Autodesk Inventor part; units mm, degrees
ref_plane "YZ Plane" through (0, 0, 0) normal (1, 0, 0) x (0, 1, 0)
ref_plane "XZ Plane" through (0, 0, 0) normal (0, 1, 0) x (-1, 0, 0)
ref_plane "XY Plane" through (0, 0, 0) normal (0, 0, 1) x (1, 0, 0)
sketch "Sketch1" plane through (0, 0, 0) normal (0, 0, 1) x (1, 0, 0)
  line L0 (-26, -31) -> (26, -31)
  line L1 (26, -31) -> (26, 31)
  line L2 (26, 31) -> (-26, 31)
  line L3 (-26, 31) -> (-26, -31)
  line L4 (-26, -31) -> (26, 31) construction
  line L5 (26, -31) -> (-26, 31) construction
  line L6 (-24, -23) -> (-24, -9) construction
  line L7 (-26, 31) -> (26, 46)
  line L8 (26, 46) -> (86, 46)
  line L9 (86, 46) -> (86, 19)
  line L10 (86, 19) -> (26, 19)
  point P0 (0, 0)
  dimension "d0" = 2
  dimension "d1" = 62
  dimension "d2" = 52
  dimension "d3" = 15
  dimension "d4" = 50
  dimension "d5" = 60
extrude "Extrusion1" add sketch "Sketch1" along normal blind 5
sketch "Sketch2" plane through (0, 0, 5) normal (0, 0, 1) x (1, 0, 0)
  line L0 (-29, 11.5) -> (-29, 6.5) construction
  line L1 (-29, 6.5) -> (-24, 6.5) construction
  line L2 (-24, 6.5) -> (-24, -20) construction
  line L3 (-24, -20) -> (-15, -20) construction
  line L4 (-15, -20) -> (-15, -27) construction
  line L5 (-15, -27) -> (-12, -27) construction
  line L6 (-12, -27) -> (-12, -20) construction
  line L7 (-12, -20) -> (16, -20) construction
  line L8 (16, -20) -> (16, 20) construction
  line L9 (16, 20) -> (11, 20) construction
  line L10 (11, 20) -> (11, 25) construction
  line L11 (11, 25) -> (8, 25) construction
  line L12 (8, 25) -> (8, 20) construction
  line L13 (8, 20) -> (-12, 20) construction
  line L14 (-12, 20) -> (-12, 27) construction
  line L15 (-12, 27) -> (-15, 27) construction
  line L16 (-15, 27) -> (-15, 20) construction
  line L17 (-15, 20) -> (-24, 20) construction
  line L18 (26, 46) -> (-26, 31)
  line L19 (-24, 20) -> (-24, 11.5) construction
  line L20 (-24, 11.5) -> (-29, 11.5) construction
  line L21 (-26, 31) -> (-26, -31) construction
  line L22 (-26, -31) -> (26, -31) construction
  line L23 (-12, 31.0385) -> (-12, 20)
  line L24 (-12, 20) -> (-8, 20)
  line L25 (-8, 20) -> (-8, 32.1923)
  line L26 (-26, 27) -> (26, 42)
  line L27 (-26, -27) -> (-12, -27)
  line L28 (-12, -27) -> (-12, -20)
  line L29 (-12, -20) -> (-8, -20)
  line L30 (-8, -20) -> (-8, -27)
  line L31 (-8, -27) -> (16, -27)
  line L32 (16, -27) -> (16, 20)
  line L33 (26, -31) -> (26, 19)
  line L34 (26, 24) -> (26, 19) construction
  line L35 (-26, 31) -> (-26, 27)
  line L36 (86, 46) -> (26, 46)
  line L37 (26, 46) -> (26, 42)
  line L38 (26, 42) -> (82, 42)
  line L39 (82, 42) -> (82, 19)
  line L40 (26, 19) -> (86, 19)
  line L41 (86, 19) -> (86, 46)
  line L42 (-26, -27) -> (-26, -31)
  line L43 (-26, -31) -> (26, -31)
  line L44 (16, 20) -> (16, 24)
  line L45 (16, 24) -> (26, 24)
  line L46 (26, 24) -> (82, 24)
  line L47 (26, 19) -> (26, 20)
  line L48 (26, 20) -> (82, 20)
  point P0 (0, 0)
  dimension "d8" = 3
  dimension "d9" = 3
  dimension "d10" = 3
  dimension "d11" = 7
  dimension "d12" = 54
  dimension "d13" = 7
  dimension "d14" = 5
  dimension "d15" = 5
  dimension "d16" = 2
  dimension "d17" = 9
  dimension "d18" = 8.5
  dimension "d19" = 4
  dimension "d20" = 5
  dimension "d21" = 5
  dimension "d22" = 40
  dimension "d23" = 4
  dimension "d25" = 4
  dimension "d26" = 10
  dimension "d27" = 4
  dimension "d28" = 4
  dimension "d36" = 1
  dimension "d37" = 4
extrude "Extrusion2" add sketch "Sketch2" along normal blind 10 contours L37 L26 L35 L18 | L36 L41 L40 L39 L38 L37 | L25 L24 L23 L26 | L39 L48 L47 L33 L43 L42 L27 L28 L29 L30 L31 L32 L44 L45 L46
sketch "Sketch3" plane through (0, 0, 15) normal (0, 0, 1) x (1, 0, 0)
  line L0 (-26, 27) -> (-12, 31.0385)
  line L1 (-12, 31.0385) -> (-12, 20)
  line L2 (-12, 20) -> (-8, 20)
  line L3 (-8, 20) -> (-8, 32.1923)
  line L4 (-8, 32.1923) -> (26, 42)
  line L5 (26, 42) -> (82, 42)
  line L6 (82, 42) -> (82, 24)
  line L7 (82, 19) -> (86, 19)
  line L8 (86, 19) -> (86, 46)
  line L9 (86, 46) -> (26, 46)
  line L10 (26, 46) -> (-26, 31)
  line L11 (-26, 31) -> (-26, 27)
  line L12 (30, 42) -> (78, 42)
  line L13 (78, 42) -> (78, 46)
  line L14 (78, 46) -> (30, 46)
  line L15 (30, 46) -> (30, 42)
  line L16 (82, 24) -> (16, 24)
  line L17 (16, 24) -> (16, -27)
  line L18 (16, -27) -> (-8, -27)
  line L19 (-8, -27) -> (-8, -20)
  line L20 (-8, -20) -> (-12, -20)
  line L21 (-12, -20) -> (-12, -27)
  line L22 (-12, -27) -> (-26, -27)
  line L23 (-26, -27) -> (-26, -31)
  line L24 (-26, -31) -> (26, -31)
  line L25 (26, -31) -> (26, 20)
  line L26 (26, 20) -> (82, 20)
  line L27 (82, 20) -> (82, 19)
  point P0 (0, 0)
  point P1 (30, 46)
  dimension "d31" = 4
  dimension "d32" = 4
extrude "Extrusion3" cut sketch "Sketch3" against normal through all contours L9 L13 L5 L15
sketch "Sketch4" plane through (26, 20, 5) normal (0, -1, 0) x (1, 0, 0)
  line L0 (0, 10) -> (56, 10)
  arc A0 (13.5, 10) -> (38.5, 10) centre (26, 10) ccw
  line L1 (0, -5) -> (0, 10)
  line L2 (13.5, 10) -> (38.5, 10)
  point P0 (-26, -5)
  dimension "d38" = 25
  dimension "d39" = 26
sketch "Sketch5" plane through (26, 19, 0) normal (0, -1, 0) x (1, 0, 0)
  line L0 (0, 0) -> (60, 0)
  line L1 (60, 0) -> (60, -7)
  line L2 (60, -7) -> (10, -7)
  line L3 (10, -7) -> (0, 0)
  point P0 (-26, 0)
  dimension "d40" = 50
  dimension "d41" = 7
extrude "Extrusion4" add sketch "Sketch5" against normal up to surface (27 mm away)
sketch "Sketch6" plane through (26, 19, 5) normal (0, -1, 0) x (1, 0, 0)
  line L0 (0, 0) -> (56, 0)
  line L1 (56, 0) -> (56, -8)
  line L2 (56, -8) -> (10, -8)
  line L3 (0, -5) -> (0, 10)
  line L4 (60, -12) -> (60, 10)
  line L5 (10, -12) -> (60, -12)
  line L6 (0, -5) -> (10, -12)
  line L7 (10, -8) -> (10, -12)
  line L8 (10, -8) -> (0, -1)
  point P0 (-26, -5)
  point P1 (35, -12)
  dimension "d44" = 4
  dimension "d45" = 4
  dimension "d47" = 4
extrude "Extrusion5" cut sketch "Sketch6" against normal up to surface (1 mm away) contours L0 L1 L2 L8 L3
extrude "Extrusion6" add sketch "Sketch4" along normal up to surface (1 mm away)
sketch "Sketch8" plane through (30, 42, 5) normal (0, 1, 0) x (1, 0, 0)
  line L0 (0, 5) -> (48, 5)
  line L1 (0, 0) -> (0, 5)
  line L2 (48, 0) -> (0, 0)
  line L3 (48, 0) -> (48, 5)
  line L4 (-14, 0) -> (52, 0)
  line L5 (2, 0) -> (10.5714, 6)
  line L6 (10.5714, 6) -> (48, 6)
  line L7 (48, 6) -> (48, 0)
  line L8 (2, 0) -> (48, 0)
  line L9 (-4, 5) -> (6, 12)
  line L10 (48, 6) -> (52, 6)
  line L11 (52, 6) -> (52, 0)
  line L12 (52, 0) -> (48, 0)
  line L13 (48, 0) -> (48, 6)
  point P0 (-30, 5)
  point P1 (9.1429, 5)
  point P2 (2, 0)
  dimension "d57" = 2
extrude "Extrusion8" cut sketch "Sketch8" against normal up to surface (18 mm away) contours L5 L6 L7 L0 | L0 L3 L2 L5 | L7 L10 L11 L4 L3
sketch "Sketch9" plane through (-26, -31, 0) normal (0, -1, 0) x (1, 0, 0)
  line L0 (62, -3) -> (52, 4)
  line L1 (52, 0) -> (52, 4)
  line L2 (52, 0) -> (62, -7)
  line L3 (62, -7) -> (112, -7)
  line L4 (112, -7) -> (112, 15)
  line L5 (108, 15) -> (112, 15)
  line L6 (108, 15) -> (108, -3)
  line L7 (108, -3) -> (62, -3)
  line L8 (52, 15) -> (65.5, 15)
  line L9 (65.5, 15) -> (90.5, 15)
  line L10 (90.5, 15) -> (108, 15)
  line L11 (0, 0) -> (52, 0)
  line L12 (52, 0) -> (52, 15)
  line L13 (0, 15) -> (52, 15)
  line L14 (0, 0) -> (0, 15)
  point P0 (26, 0)
extrude "Extrusion9" add sketch "Sketch9" along normal blind 15
sketch "Sketch10" plane through (0, 0, 15) normal (0, 0, 1) x (1, 0, 0)
  line L0 (26, -31) -> (86, -31)
  line L1 (86, -31) -> (86, -38)
  line L2 (86, -38) -> (26, -38)
  line L3 (26, -38) -> (26, -31)
  point P0 (0, 0)
  dimension "d62" = 7
extrude "Extrusion10" cut sketch "Sketch10" against normal through all
sketch "Sketch11" plane through (0, 0, 15) normal (0, 0, 1) x (1, 0, 0)
  line L0 (-26, -46) -> (26, -46)
  line L1 (26, -46) -> (-26, -46)
  line L2 (-26, -46) -> (-26, -36.5)
  line L3 (26, -46) -> (-26, -36.5)
  point P0 (0, 0)
  dimension "d65" = 9.5
extrude "Extrusion11" cut sketch "Sketch11" against normal through all
sketch "Sketch12" plane through (26, -38, 15) normal (0, 1, 0) x (1, 0, 0)
  arc A0 (38.5, 0) -> (13.5, 0) centre (26, 0) ccw
  line L0 (13.5, 0) -> (38.5, 0)
  circle A1 centre (26, 0) radius 2.5
  point P0 (-26, 15)
  dimension "d68" = 5
extrude "Extrusion12" cut sketch "Sketch12" against normal through all contours A1 L0 | L0 A1
properties part number "wirst 1 left"
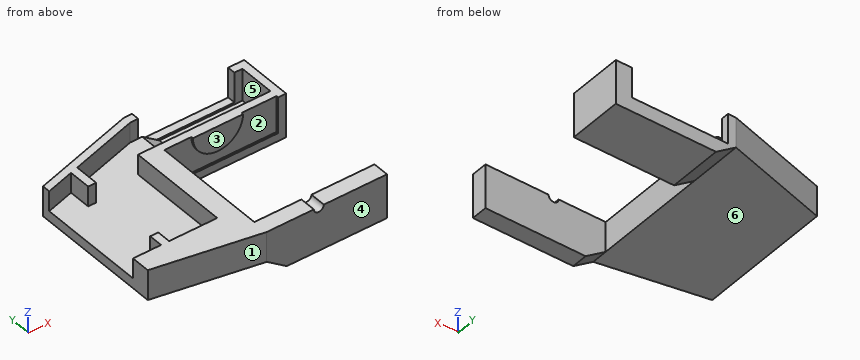
Work out the finished part from the listing and answer in its coordinate system (mm). Face numbers are marked on the shaded views. A direction names the side the tool comes from. Coordinates: 2 decimals unless noted, no trailing zeros. Loops run counter-clockwise (first coordinate to the right, second up) from the corner with the lowest first, then second, coordinate; pieces in that order, holes last.
1) Consider probe 1 along Y at (x, z) = (59.5, 1.25); probe 2 along Y at (x, z) = (50, 8.5); probe 3 along X at (y, z) = (-23.5, 7.75). Determine where each line is inside the solid, lowest interval first.
Results:
probe 1: y = -46 to -38, 20 to 24
probe 2: y = -46 to -38, 19 to 24
probe 3: x = -12 to -8, 16 to 26
2) Flat-ended cylindrical pins translate along their axes: pin 1 (10 mm diameter, centred on x = 12.5, z = 8.5, fed in from +Y); pin 2 (3.5 mm diameter, centred on y = -22, z = 8.5, fed in from -X); pin 3 (2 mm diameter, centred on x = 11, y = -13.5, fed in from +Z). Find the tip coordinate at first contact, or state that the pin passes through.
Results:
pin 1: stops at y = 43.55
pin 2: stops at x = -12
pin 3: stops at z = 5
3) Section C-C (y = 40) is taken. Give the vertices of the cut face in (x, z).
Results:
outline: (5.2, 0) - (26, 0) - (36, -7) - (86, -7) - (86, 15) - (82, 15) - (82, -1) - (40.57, -1) - (32, 5) - (19.07, 5) - (19.07, 15) - (5.2, 15) - close
4) For a pull along Y with two mould halves and no side action, classify the marked faces 4, 5 and 6 as +Y half, -Y half, draft (parallel to the pull), parting line (faces both ways), or undercut.
Results:
face 4: -Y half
face 5: undercut
face 6: draft
5) Section B-B (y = 12) is taken. Give the vertices of the cut face in (x, z).
Results:
outline: (-26, 0) - (26, 0) - (26, 15) - (16, 15) - (16, 5) - (-26, 5) - close
6) For the marked faces 1, 2 and 3, determine the directions among +Z, -Z, +X, -X, +Y, -Y from which every point of the face is accessible in a straight line to the end or side of a thin tool.
Results:
face 1: +Z, -Z, -X, -Y
face 2: none
face 3: +Z, -Z, +X
7) Section D-D (y = -33) is taken. Give the vertices of the cut face in (x, z), plus the area to 3 significant figures.
Results:
outline: (-26, 0) - (26, 0) - (26, 15) - (-26, 15) - close
area: 780 mm2
8) Section A-A (x = 52) is taken. Give the vertices of the cut face in (y, z), plus the area to 4 significant figures.
Results:
outline: (-46, -7) - (-38, -7) - (-38, 12.5) - (-46, 12.5) - close; (19, -7) - (46, -7) - (46, 0) - (42, 0) - (42, -1) - (24, -1) - (24, 15) - (19, 15) - (19, 2.5) - (20, 2.5) - (20, -3) - (19, -3) - close
area: 396.5 mm2
